from build123d import *

# Parameters (mm, degrees)
SKETCH2_W           = 35
SKETCH2_H           = 35
BOSS_EXTRUDE1_DEPTH = 3
SKETCH3_W           = 20
SKETCH3_H           = 8
BOSS_EXTRUDE2_DEPTH = 2


with BuildPart() as part:
    # Sketch2 → Boss-Extrude1 (new body)
    with BuildSketch(Plane.XY):
        Rectangle(SKETCH2_W, SKETCH2_H)
    extrude(amount=BOSS_EXTRUDE1_DEPTH)

    # Sketch3 → Boss-Extrude2 (add)
    with BuildSketch(Plane.XY.offset(3)):
        with BuildLine():
            Line((-13.2, 8.25), (-13.2, 11.75))
            ThreePointArc((-13.2, 11.75), (-12, 12.95), (-10.8, 11.75))
            Line((-10.8, 11.75), (-10.8, 8.25))
            ThreePointArc((-10.8, 8.25), (-12, 7.05), (-13.2, 8.25))
        make_face()
        with BuildLine():
            Line((-13.2, -11.75), (-13.2, -8.25))
            ThreePointArc((-13.2, -8.25), (-12, -7.05), (-10.8, -8.25))
            Line((-10.8, -8.25), (-10.8, -11.75))
            ThreePointArc((-10.8, -11.75), (-12, -12.95), (-13.2, -11.75))
        make_face()
        with BuildLine():
            Line((10.8, -11.75), (10.8, -8.25))
            ThreePointArc((10.8, -8.25), (12, -7.05), (13.2, -8.25))
            Line((13.2, -8.25), (13.2, -11.75))
            ThreePointArc((13.2, -11.75), (12, -12.95), (10.8, -11.75))
        make_face()
        with BuildLine():
            Line((10.8, 8.25), (10.8, 11.75))
            ThreePointArc((10.8, 11.75), (12, 12.95), (13.2, 11.75))
            Line((13.2, 11.75), (13.2, 8.25))
            ThreePointArc((13.2, 8.25), (12, 7.05), (10.8, 8.25))
        make_face()
        with Locations((0, 10)):
            Rectangle(SKETCH3_W, SKETCH3_H)
    extrude(amount=BOSS_EXTRUDE2_DEPTH)


solid = part.part
Build history of the part. All positions in model axes, mm. A direction names the side the tool comes from. Round coordinates to 2 decimals unless told otherwise and drop trailing zeros. Loops run counter-clockwise (first coordinate to the right, second up) from the corner with the lowest first, then second, coordinate; pieces in that order, holes last. Notation, with made-up numbers: (30, -35) -> (50, -35) arc R21 cw to (50, -25) -> close; hole circle Ø1 at (-6.5, 69). An arc over 180 degrees is marked (long way). One line per item, written item: value. Start each with the question number.
Q1. Drop flat-ended pins along their axis: pin 1 Ø0.6 at (y, z) = (-9.5, 4) entering from +X; pin 2 Ø1 at (x, z) = (-2.5, 4.5) entering from -Y; pin 3 Ø0.6 at (y, z) = (10, 4) entering from -X. Give the stop position or say it passes through.
Q2. 3-axis set-ups, long thin cutter, end or side, ignore diameter. For faces 1 (the face through (-12.03, -7.05, 3.99)), 2 (the face through (12.03, -12.95, 3.99)), 3 (the face through (-12.03, 12.95, 3.99)): which of +Z, -Z, +X, -X, +Y, -Y reach the whole face in a straight line?
Q3. Cut at A-A on x = -12. List the corners of the cut face in (y, z).
Q4. Cut at B-B on y = -5. List the corners of the cut face in (x, z).
Q5. Two-plate mould, pull along X, no slides. Class faces 4 (the face through (-12, 10, 5)), 5 (the face through (-13.2, -10, 4)), 6 (the face through (12.03, 7.05, 3.99)): released by +X, released by -X, zero draft, split by the parting line, or undercut.
Q6. Cut at C-C on x = -6. List the corners of the cut face in (y, z).
Q7. Probe line 1 along X through (y, z) = (12, 4.2); line 2 along Z through (x, y) = (4.5, 3). List the from-to ranges inside material, lowest first.
Computed:
1. pin 1: x = 13.2
1. pin 2: y = 6
1. pin 3: x = -13.2
2. face 1: +Z
2. face 2: +Z, -Y
2. face 3: +Z, +Y
3. outline: (-17.5, 0) -> (17.5, 0) -> (17.5, 3) -> (12.95, 3) -> (12.95, 5) -> (7.05, 5) -> (7.05, 3) -> (-7.05, 3) -> (-7.05, 5) -> (-12.95, 5) -> (-12.95, 3) -> (-17.5, 3) -> close
4. outline: (-17.5, 0) -> (17.5, 0) -> (17.5, 3) -> (-17.5, 3) -> close
5. face 4: zero draft
5. face 5: released by -X
5. face 6: undercut
6. outline: (-17.5, 0) -> (17.5, 0) -> (17.5, 3) -> (14, 3) -> (14, 5) -> (6, 5) -> (6, 3) -> (-17.5, 3) -> close
7. line 1: -13.17 to -10.83, -10 to 10, 10.83 to 13.17
7. line 2: 0 to 3
